Verification items for the finished model (mm, model axes). A direction names the side the tool comes from. Give positions to 0.01 mm unless a question says otherwise; leave off trailing zeros. Order: outer loops, then holes, each group sorted by start corner. A loop starts at its lowest first (then second) coordinate and runs counter-clockwise, first axis right, second up.
(1) Sectioned sample at A-A on z = 0. Count the separate pieces of the cut face and the enclosed holes in it, plus the area to 3 significant figures.
(2) Scan lines: L1, parallel to Z at x = -19.05, y = 6.75 (3 decimals); L2, parallel to X at y = 1.7, z = 0; L3, parallel to Z at x = 1.5, y = 10.75. Record each from-to range of solid material in increasing order.
(3) Gauge pin test, flat ends, axial feed: pin 1 (5 mm diameter, centred on x = -16, z = -0.5, fed in from +Y); pin 2 (4.5 mm diameter, centred on x = 0, z = 16.51, fed in from +Y); pin 3 (10 mm diameter, centred on x = -1.5, z = 18, fed in from -Y); pin 4 (6 mm diameter, centred on x = 0, z = -16.51, fed in from -Y) (3 decimals). Record the tip position at first contact, or that the pin passes through.
(4) Sectioned sample at D-D on y = 12.5. Record the cut outline in (x, z) (3 decimals).
(5) Mould release check, pull along X, two halves, no side actions. Record for faces 6 (the face through (0, 15.875, 0)), 7 (the face through (25.4, 8, 0)), 8 (the face through (-20.609, 7.826, -16.053)): pulls with the +X half, pulls with the -X half, needs draft (parallel to the pull), parting line crosses it, or undercut.
(6) Access from +Z, -Z, +X, -X, +Y, -Y to the whole of each face (thin tool, end or side, straight path). Record for faces 1 (the face through (-5, 11, -6.35)), 2 (the face through (0, 9.525, 22)), 3 (the face through (4.18, 11.65, 16.01)), 4 (the face through (-0.794, 12, -22)), 5 (the face through (-12, 13.97, 0)).
```python
from build123d import *

# Parameters (mm, degrees)
SKETCH1_W               = 50.8
SKETCH1_H               = 50.8
BOSS_EXTRUDE1_DEPTH     = 15.875
F_1_4_CLEARANCE_HOLE1_D = 6.7564
SKETCH7_R               = 3.175
CUT_EXTRUDE2_DEPTH      = 9.525
F_6_CLEARANCE_HOLE1_D   = 3.7973
SKETCH15_R              = 6.35
CUT_EXTRUDE5_DEPTH      = 3.175
SKETCH17_R              = 0.79375
CUT_EXTRUDE7_DEPTH      = 19.05
SKETCH19_R              = 0.79375
CUT_EXTRUDE8_DEPTH      = 19.05
SKETCH20_W              = 1.5875
SKETCH20_H              = 8.919384601
SKETCH20_W_2            = 8.609080127
SKETCH20_H_2            = 1.5875
SKETCH20_W_3            = 9.022819426
SKETCH20_H_3            = 8.367732203
CUT_EXTRUDE9_DEPTH      = 6.35
SKETCH21_R              = 9.525
CUT_EXTRUDE10_DEPTH     = 1.905


with BuildPart() as part:
    # Sketch1 → Boss-Extrude1 (new body)
    with BuildSketch(Plane(origin=(0, 0, 0), x_dir=(1, 0, 0), z_dir=(0, 1, 0))):
        Rectangle(SKETCH1_W, SKETCH1_H)
    extrude(amount=BOSS_EXTRUDE1_DEPTH)

    # 1/4 Clearance Hole1 (through all)
    with Locations(Plane(origin=(0, 15.875, 0), x_dir=(1, 0, 0), z_dir=(0, 1, 0))):
        with Locations((-19.05, -19.05), (-19.05, 19.05), (19.05, 19.05), (19.05, -19.05)):
            Hole(F_1_4_CLEARANCE_HOLE1_D / 2)

    # Sketch7 → Cut-Extrude2 (cut)
    with BuildSketch(Plane(origin=(0, 15.875, 0), x_dir=(1, 0, 0), z_dir=(0, 1, 0))):
        with Locations(Location((-16.51, 0, 0), (0, 0, 270))):
            Circle(SKETCH7_R)
        with Locations(Location((0, 16.51, 0), (0, 0, 270))):
            Circle(SKETCH7_R)
        with Locations(Location((16.51, 0, 0), (0, 0, 270))):
            Circle(SKETCH7_R)
        with Locations(Location((0, -16.51, 0), (0, 0, 270))):
            Circle(SKETCH7_R)
    extrude(amount=-CUT_EXTRUDE2_DEPTH, mode=Mode.SUBTRACT)

    # #6 Clearance Hole1 (through all)
    with Locations(Plane(origin=(0, 6.35, 0), x_dir=(1, 0, 0), z_dir=(0, 1, 0))):
        with Locations((-16.51, 0), (0, 16.51), (16.51, 0), (0, -16.51)):
            Hole(F_6_CLEARANCE_HOLE1_D / 2)

    # Sketch15 → Cut-Extrude5 (cut)
    with BuildSketch(Plane.XZ):
        with Locations(Location((0, 16.51, 0), (0, 0, 270))):
            Circle(SKETCH15_R)
        with Locations(Location((16.51, 0, 0), (0, 0, 270))):
            Circle(SKETCH15_R)
        with Locations(Location((0, -16.51, 0), (0, 0, 270))):
            Circle(SKETCH15_R)
        with Locations(Location((-16.51, 0, 0), (0, 0, 270))):
            Circle(SKETCH15_R)
    extrude(amount=-CUT_EXTRUDE5_DEPTH, mode=Mode.SUBTRACT)

    # Sketch17 → Cut-Extrude7 (cut)
    with BuildSketch(Plane.XY.offset(25.4)):
        with Locations((4.7625, 11.1125)):
            Circle(SKETCH17_R)
    extrude(amount=-CUT_EXTRUDE7_DEPTH, mode=Mode.SUBTRACT)

    # Sketch19 → Cut-Extrude8 (cut)
    with BuildSketch(Plane(origin=(0, 0, -25.4), x_dir=(-1, 0, 0), z_dir=(0, 0, -1))):
        with Locations((4.7625, 11.1125)):
            Circle(SKETCH19_R)
    extrude(amount=-CUT_EXTRUDE8_DEPTH, mode=Mode.SUBTRACT)

    # Sketch20 → Cut-Extrude9 (cut)
    with BuildSketch(Plane(origin=(0, 15.875, 0), x_dir=(1, 0, 0), z_dir=(0, 1, 0))):
        with Locations((0, 20.9403077)):
            Rectangle(SKETCH20_W, SKETCH20_H)
        with Locations((-21.095459936, 0)):
            Rectangle(SKETCH20_W_2, SKETCH20_H_2)
        with Locations((20.888590287, 0)):
            Rectangle(SKETCH20_W_3, SKETCH20_H_2)
        with Locations((0, -21.216133899)):
            Rectangle(SKETCH20_W, SKETCH20_H_3)
    extrude(amount=-CUT_EXTRUDE9_DEPTH, mode=Mode.SUBTRACT)

    # Sketch21 → Cut-Extrude10 (cut)
    with BuildSketch(Plane(origin=(0, 15.875, 0), x_dir=(1, 0, 0), z_dir=(0, 1, 0))):
        with Locations((-16.51, 0)):
            Circle(SKETCH21_R)
        with Locations((16.51, 0)):
            Circle(SKETCH21_R)
        with Locations((0, 16.51)):
            Circle(SKETCH21_R)
        with Locations((0, -16.51)):
            Circle(SKETCH21_R)
    extrude(amount=-CUT_EXTRUDE10_DEPTH, mode=Mode.SUBTRACT)


solid = part.part
```
Ans:
1. separate pieces: 3
1. enclosed holes: 0
1. area: 484 mm2
2. L1: z = -25.4 to -22.428, -15.672 to -1.905, 1.905 to 15.672, 22.428 to 25.4
2. L2: x = -25.4 to -22.86, -10.16 to 10.16, 22.86 to 25.4
2. L3: z = -25.4 to -19.31, -13.71 to 13.71, 19.31 to 25.4
3. pin 1: stops at y = 13.97
3. pin 2: stops at y = 6.35
3. pin 3: stops at y = 0
3. pin 4: stops at y = 3.175
4. outline: (-25.4, -25.4) - (-0.794, -25.4) - (-0.794, -19.584) arc R3.175 cw (long way) to (0.794, -19.584) - (0.794, -25.4) - (25.4, -25.4) - (25.4, -0.794) - (19.584, -0.794) arc R3.175 cw (long way) to (19.584, 0.794) - (25.4, 0.794) - (25.4, 25.4) - (0.794, 25.4) - (0.794, 19.584) arc R3.175 cw (long way) to (-0.794, 19.584) - (-0.794, 25.4) - (-25.4, 25.4) - (-25.4, 0.794) - (-19.584, 0.794) arc R3.175 cw (long way) to (-19.584, -0.794) - (-25.4, -0.794) - close; hole circle Ø6.756 at (-19.05, -19.05); hole circle Ø6.756 at (-19.05, 19.05); hole circle Ø6.756 at (19.05, -19.05); hole circle Ø6.756 at (19.05, 19.05)
5. face 6: needs draft
5. face 7: pulls with the +X half
5. face 8: undercut
6. face 1: -Z
6. face 2: +Z, +Y
6. face 3: +Z
6. face 4: -Z, +Y
6. face 5: +Y
